Here's how the part is built. I have some questions about the finished solid (model axes, mm). A direction names the side the tool comes from. Round coordinates to 2 decimals unless told otherwise and drop trailing zeros. Loops run counter-clockwise (first coordinate to the right, second up) from the corner with the lowest first, then second, coordinate; pieces in that order, holes last. Notation, with made-up numbers: (82, -31) -> (92, -31) arc R11 cw to (92, -17) -> close; hole circle Ø9 at (-6.5, 35). An arc over 180 degrees is marked (long way). Use one line per item in the form item = value. Start each with the question number.
Item 1: If I drill on L1, parallel to Z at x = -123.5, y = 20.25 (3 decimals); L2, parallel to Z at x = -80, y = 23.25 (3 decimals); L3, parallel to X at y = 10.25, z = 7.5 (3 decimals), over which ranges is the centre line in solid material (lowest first)? Write a range as [from, to].
Item 2: Thinking about a two-plate mould opening in Z: for faces 1 (the face through (-108, 13, 0)), 2 (the face through (-152.4, 13, 75)), 3 (the face through (-151, 13, 73.025)), which applies, released by +Z, released by -Z, zero draft, split by the parting line, or undercut?
Item 3: I'm going to push flat-ended pins straight in: pin 1 Ø1 at (x, y) = (-151, 17) entering from -Z (3 decimals); pin 2 Ø1.6 at (x, y) = (-1, 11) entering from +Z (3 decimals); pin 3 Ø12 at (x, z) = (-45, 39) entering from -Y; pin 4 Ø1 at (y, z) = (10.5, 2.5) entering from -X. Where does each tip first touch, or does it pass through?
Item 4: If we section it at B-B (z = 12): Write out the boundary of the cut face in (x, y) (3 decimals).
Item 5: If we section it at A-A (x = -99): Write out the boundary of the cut face in (y, z) (3 decimals).
Item 6: For faces 4 (the face through (-151, 13, 15.875)), 5 (the face through (-2, 13, 31.75)), 6 (the face through (-50.8, 13, 2)), which set-ups out of +Z, -Z, +X, -X, +Y, -Y let a thin tool reach every point of the face, with its end or its side?
Autodesk Inventor part; units mm, degrees
ref_plane "YZ Plane" through (0, 0, 0) normal (1, 0, 0) x (0, 1, 0)
ref_plane "XZ Plane" through (0, 0, 0) normal (0, 1, 0) x (-1, 0, 0)
ref_plane "XY Plane" through (0, 0, 0) normal (0, 0, 1) x (1, 0, 0)
sketch "Sketch1" plane through (0, 0, 0) normal (0, 1, 0) x (-1, 0, 0)
  line L0 (0, 0) -> (0, 76.2)
  line L1 (0, 76.2) -> (152.4, 76.2)
  line L2 (152.4, 76.2) -> (152.4, 0)
  line L3 (152.4, 0) -> (0, 0)
  line L4 (139.7, 76.2) -> (127, 76.2)
  line L5 (127, 76.2) -> (127, 73.025)
  line L6 (127, 73.025) -> (139.7, 73.025)
  line L7 (139.7, 73.025) -> (139.7, 76.2)
  line L8 (114.3, 76.2) -> (101.6, 76.2)
  line L9 (101.6, 76.2) -> (101.6, 73.025)
  line L10 (101.6, 73.025) -> (114.3, 73.025)
  line L11 (114.3, 73.025) -> (114.3, 76.2)
  line L12 (88.9, 76.2) -> (76.2, 76.2)
  line L13 (76.2, 76.2) -> (76.2, 73.025)
  line L14 (76.2, 73.025) -> (88.9, 73.025)
  line L15 (88.9, 73.025) -> (88.9, 76.2)
  line L16 (63.5, 76.2) -> (50.8, 76.2)
  line L17 (50.8, 76.2) -> (50.8, 73.025)
  line L18 (50.8, 73.025) -> (63.5, 73.025)
  line L19 (63.5, 73.025) -> (63.5, 76.2)
  line L20 (38.1, 76.2) -> (25.4, 76.2)
  line L21 (25.4, 76.2) -> (25.4, 73.025)
  line L22 (25.4, 73.025) -> (38.1, 73.025)
  line L23 (38.1, 73.025) -> (38.1, 76.2)
  line L24 (12.7, 76.2) -> (0, 76.2)
  line L25 (0, 76.2) -> (0, 73.025)
  line L26 (0, 73.025) -> (12.7, 73.025)
  line L27 (12.7, 73.025) -> (12.7, 76.2)
  line L28 (152.4, 0) -> (139.7, 0)
  line L29 (139.7, 0) -> (139.7, 3.175)
  line L30 (139.7, 3.175) -> (152.4, 3.175)
  line L31 (152.4, 3.175) -> (152.4, 0)
  line L32 (127, 0) -> (114.3, 0)
  line L33 (114.3, 0) -> (114.3, 3.175)
  line L34 (114.3, 3.175) -> (127, 3.175)
  line L35 (127, 3.175) -> (127, 0)
  line L36 (101.6, 0) -> (88.9, 0)
  line L37 (88.9, 0) -> (88.9, 3.175)
  line L38 (88.9, 3.175) -> (101.6, 3.175)
  line L39 (101.6, 3.175) -> (101.6, 0)
  line L40 (76.2, 0) -> (63.5, 0)
  line L41 (63.5, 0) -> (63.5, 3.175)
  line L42 (63.5, 3.175) -> (76.2, 3.175)
  line L43 (76.2, 3.175) -> (76.2, 0)
  line L44 (50.8, 0) -> (38.1, 0)
  line L45 (38.1, 0) -> (38.1, 3.175)
  line L46 (38.1, 3.175) -> (50.8, 3.175)
  line L47 (50.8, 3.175) -> (50.8, 0)
  line L48 (25.4, 0) -> (12.7, 0)
  line L49 (12.7, 0) -> (12.7, 3.175)
  line L50 (12.7, 3.175) -> (25.4, 3.175)
  line L51 (25.4, 3.175) -> (25.4, 0)
  line L52 (152.4, 73.025) -> (149.225, 73.025)
  line L53 (149.225, 73.025) -> (149.225, 60.325)
  line L54 (149.225, 60.325) -> (152.4, 60.325)
  line L55 (152.4, 60.325) -> (152.4, 73.025)
  line L56 (152.4, 44.45) -> (149.225, 44.45)
  line L57 (149.225, 44.45) -> (149.225, 31.75)
  line L58 (149.225, 31.75) -> (152.4, 31.75)
  line L59 (152.4, 31.75) -> (152.4, 44.45)
  line L60 (152.4, 15.875) -> (149.225, 15.875)
  line L61 (149.225, 15.875) -> (149.225, 3.175)
  line L62 (149.225, 3.175) -> (152.4, 3.175)
  line L63 (152.4, 3.175) -> (152.4, 15.875)
  line L64 (0, 73.025) -> (0, 60.325)
  line L65 (0, 60.325) -> (3.175, 60.325)
  line L66 (3.175, 60.325) -> (3.175, 73.025)
  line L67 (3.175, 73.025) -> (0, 73.025)
  line L68 (0, 3.175) -> (0, 15.875)
  line L69 (0, 15.875) -> (3.175, 15.875)
  line L70 (3.175, 15.875) -> (3.175, 3.175)
  line L71 (3.175, 3.175) -> (0, 3.175)
  line L72 (0, 31.75) -> (0, 44.45)
  line L73 (0, 44.45) -> (3.175, 44.45)
  line L74 (3.175, 44.45) -> (3.175, 31.75)
  line L75 (3.175, 31.75) -> (0, 31.75)
  point P0 (149.225, 3.175)
  dimension "d176" = 76.2
  dimension "d177" = 152.4
  dimension "d178" = 12.7
  dimension "d179" = 3.175
  dimension "d180" = 12.7
  dimension "d181" = 12.7
  dimension "d182" = 3.175
  dimension "d183" = 12.7
  dimension "d184" = 3.175
  dimension "d185" = 12.7
  dimension "d186" = 3.175
  dimension "d187" = 12.7
  dimension "d188" = 3.175
  dimension "d189" = 12.7
  dimension "d190" = 12.7
  dimension "d191" = 12.7
  dimension "d192" = 12.7
  dimension "d193" = 12.7
  dimension "d194" = 3.175
  dimension "d195" = 12.7
  dimension "d196" = 12.7
  dimension "d197" = 3.175
  dimension "d198" = 12.7
  dimension "d199" = 3.175
  dimension "d200" = 12.7
  dimension "d201" = 3.175
  dimension "d202" = 12.7
  dimension "d203" = 3.175
  dimension "d204" = 12.7
  dimension "d205" = 12.7
  dimension "d206" = 12.7
  dimension "d207" = 12.7
  dimension "d208" = 3.175
  dimension "d209" = 12.7
  dimension "d210" = 3.175
  dimension "d211" = 12.7
  dimension "d212" = 12.7
  dimension "d213" = 3.175
  dimension "d214" = 12.7
  dimension "d215" = 3.175
  dimension "d216" = 3.175
  dimension "d217" = 12.7
  dimension "d218" = 15.875
  dimension "d219" = 3.175
  dimension "d220" = 12.7
  dimension "d222" = 3.175
  dimension "d223" = 12.7
  dimension "d224" = 3.175
  dimension "d225" = 12.7
  dimension "d226" = 3.175
  dimension "d227" = 3.175
  dimension "d228" = 12.7
  dimension "d229" = 3.175
  dimension "d230" = 15.875
extrude "Extrusion5" add sketch "Sketch1" along normal blind 25.4 contours L0 L71 L70 L69 L75 L74 L73 L65 L66 L26 L27 L1 L21 L22 L23 L17 L18 L19 L13 L14 L15 L9 L10 L11 L5 L6 L7 L2 L52 L53 L54 L56 L57 L58 L60 L61 L30 L29 L3 L35 L34 L33 L39 L38 L37 L43 L42 L41 L47 L46 L45 L51 L50 L49
properties part number "BackPanel"
Values found:
q1.L1 = [3.175, 76.2]
q1.L2 = [0, 73.025]
q1.L3 = [-149.225, -3.175]
q2.face_1 = released by -Z
q2.face_2 = zero draft
q2.face_3 = undercut
q3.pin_1 = 15.875
q3.pin_2 = 60.325
q3.pin_3 = 0
q3.pin_4 = -139.7
q4.outline = (-149.225, 0) -> (-3.175, 0) -> (-3.175, 25.4) -> (-149.225, 25.4) -> close
q5.outline = (0, 3.175) -> (25.4, 3.175) -> (25.4, 76.2) -> (0, 76.2) -> close
q6.face_4 = -Z, -X, +Y, -Y
q6.face_5 = +X, +Y, -Y
q6.face_6 = -Z, +Y, -Y
